Part model, mm, in its own coordinate system. Round coordinates to 2 decimals unless told otherwise and drop trailing zeros. Loops run counter-clockwise (first coordinate to the right, second up) from the corner with the lowest first, then second, coordinate; pieces in that order, holes last. Notation, with made-up numbers: (54, 66) - (100, 66) arc R7 cw to (100, 79) - close; hole circle Ø8 at (68, 0). An arc over 180 degrees is marked (long way). Put each result on its own line as item: value.
from build123d import *

# Parameters (mm, degrees)
F0_R     = 27
F0_R_2   = 21.97
F1_DEPTH = 29
F2_SIZE2 = 0.5773502692
F2_SIZE  = 1
F3_SIZE2 = 0.2886751346
F3_SIZE  = 0.5


with BuildPart() as f1:
    # F0 (on Top) → F1 (new body)
    with BuildSketch(Plane.XY):
        Circle(F0_R)
        Circle(F0_R_2, mode=Mode.SUBTRACT)
    extrude(amount=F1_DEPTH)

    # F2
    f2_edges = [f1.edges().sort_by_distance(p)[0] for p in [
        (-21.97, 0, 29),
        (-21.97, 0, 0),
    ]]
    f2_side = f1.faces().sort_by_distance((-21.97, 0, 14.5))[0]
    chamfer(f2_edges, length=F2_SIZE, length2=F2_SIZE2, reference=f2_side)

    # F3
    f3_edges = [f1.edges().sort_by_distance(p)[0] for p in [
        (-27, 0, 29),
        (-27, 0, 0),
    ]]
    f3_side = f1.faces().sort_by_distance((-27, 0, 14.5))[0]
    chamfer(f3_edges, length=F3_SIZE, length2=F3_SIZE2, reference=f3_side)


solid = f1.part
1. Band-saw the part on A-A (x = 0). List the corners of the cut face in (y, z).
A:
outline: (-27, 0.5) - (-26.71, 0) - (-22.55, 0) - (-21.97, 1) - (-21.97, 28) - (-22.55, 29) - (-26.71, 29) - (-27, 28.5) - close; (21.97, 1) - (22.55, 0) - (26.71, 0) - (27, 0.5) - (27, 28.5) - (26.71, 29) - (22.55, 29) - (21.97, 28) - close
2. Pin check, flat tips, straight feed: P1, Ø5, axis at x = 17.5, z = 21, coming from the -Y side; P2, Ø6, axis at x = -6.5, z = 5, coming from the +Y side; P3, Ø1.5, axis at y = -15.5, z = 22.5, coming from the +X side (3 decimals). Stop position of each tip, or through.
A:
P1: stops at y = -22.45
P2: stops at y = 26.77
P3: stops at x = 22.615
3. Band-saw the part on C-C (z = 14). List the corners of the cut face in (x, y).
A:
outline: circle Ø54 at (0, 0); hole circle Ø43.94 at (0, 0)
4. Probe line 1 along Y through (x, z) = (0, 19.5); line 2 along Y through (x, z) = (-20, 12); line 3 along X through (y, z) = (-19, 21.75). List the from-to ranges inside material, lowest first. Write a range as [from, to].
A:
line 1: y = [-27, -21.97], [21.97, 27]
line 2: y = [-18.14, -9.09], [9.09, 18.14]
line 3: x = [-19.18, -11.03], [11.03, 19.18]
